Geometry: see drawing. Coordinates: mm, zero at the bounding-box minimum. A direction names the side the tool comes from. Round coordinates to 2 decimals unless told otherwise and drop trailing zeros. Write each loop counter-clockwise with the first axis right and the second up, starting at its lowest first coordinate (ties: lowest second). Pieces come first, ordered by that corner, then holes. Notation, with made-up numbers: M -29.75,39 L -22.75,39 A21 cw -22.75,76 Z; hole C -29,12 d10. An arc over 180 degrees is marked long. Use a Markdown table: item, result.
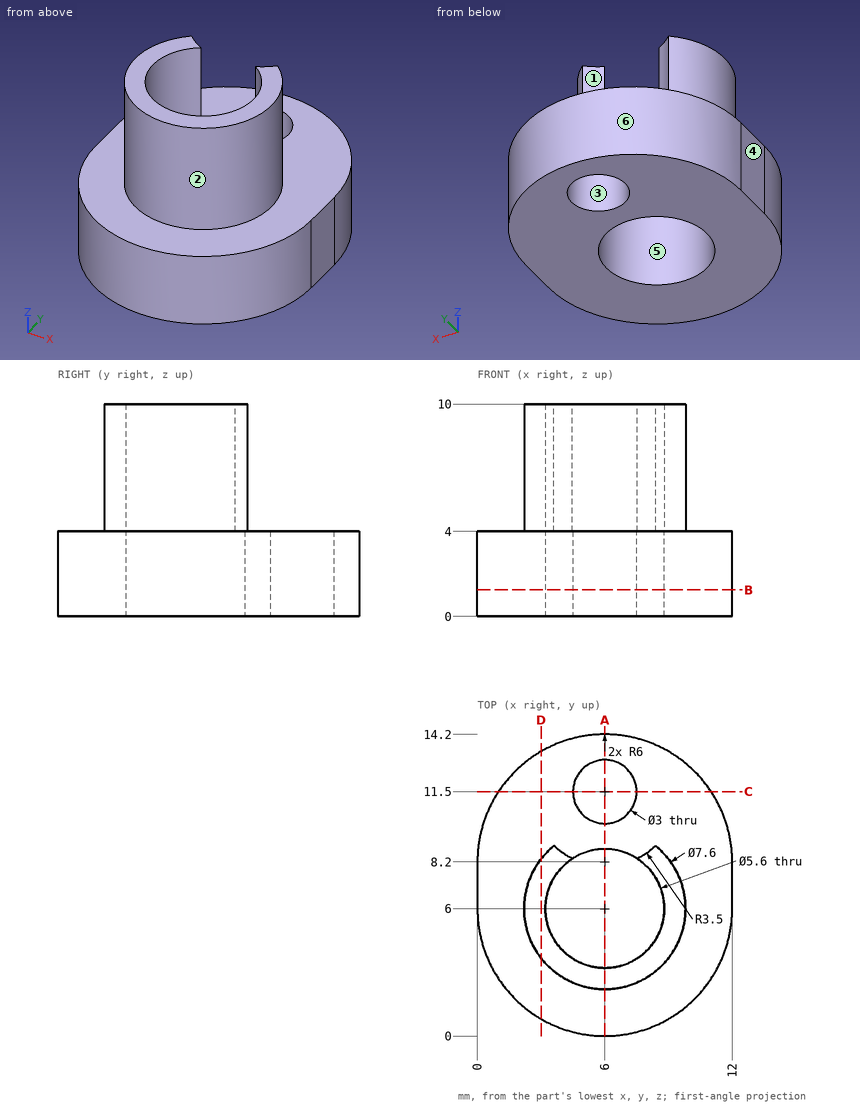
Q1. Section C-C on y = 11.5. Return loops of the section in (x, z).
Results are:
| item | result |
|---|---|
| outline | M 0.99,0 L 4.5,0 L 4.5,4 L 0.99,4 Z; M 7.5,0 L 11.01,0 L 11.01,4 L 7.5,4 Z |
Q2. Section B-B on z = 1.25. Return loops of the section in (x, y).
Results are:
| item | result |
|---|---|
| outline | M 0,6 A6 ccw 12,6 L 12,8.2 A6 ccw 0,8.2 Z; hole C 6,6 d5.6; hole C 6,11.5 d3 |
Q3. Reachability of the marked faces 1, 2 and 3 from +Z, -Z, +X, -X, +Y, -Y: full face, straight path, thin tool, end or side. Return the list, or none.
Results are:
| item | result |
|---|---|
| face 1 | +Z, +Y |
| face 2 | +Z |
| face 3 | +Z, -Z |
Q4. Mould query, pull axis X, two halves, no side actions, for the marked faces 4, 5 and 6. Classes: +X half, -X half, draft (parallel to the pull), parting line (faces both ways), or undercut.
Results are:
| item | result |
|---|---|
| face 4 | -X half |
| face 5 | undercut |
| face 6 | parting line |
Q5. Section D-D on x = 3. Return loops of the section in (y, z), plus the area to 3 significant figures.
Results are:
| item | result |
|---|---|
| outline | M 0.8,0 L 13.4,0 L 13.4,4 L 8.33,4 L 8.33,10 L 3.67,10 L 3.67,4 L 0.8,4 Z |
| area | 78.4 mm^2 |
Q6. Section A-A on x = 6. Return loops of the section in (y, z).
Results are:
| item | result |
|---|---|
| outline | M 0,0 L 3.2,0 L 3.2,10 L 2.2,10 L 2.2,4 L 0,4 Z; M 8.8,0 L 10,0 L 10,4 L 8.8,4 Z; M 13,0 L 14.2,0 L 14.2,4 L 13,4 Z |
Q7. First-contact query: pin 1 Ø6 at (x, y) = (3.5, 2.5) entering from -Z; pin 2 Ø5 at (x, z) = (8.5, 5.5) entering from -Y; pin 3 Ø2 at (x, z) = (7, 6) entering from +Y; pin 4 Ø3 at (x, z) = (8.5, 1.5) entering from -Y. Flat tips, straight axial feed; report the tip coordinate or a pass-through.
Results are:
| item | result |
|---|---|
| pin 1 | z = 0 |
| pin 2 | y = 0.02 |
| pin 3 | y = 8.63 |
| pin 4 | y = 0.08 |
Q8. Line query: L1, parallel to Y at x = 6, z = 2.75; L2, parallel to X at y = 6, z = 5; L3, parallel to Y at x = 6, z = 7.75. Output: solid intervals per line, ascending.
Results are:
| item | result |
|---|---|
| L1 | 0 to 3.2, 8.8 to 10, 13 to 14.2 |
| L2 | 2.2 to 3.2, 8.8 to 9.8 |
| L3 | 2.2 to 3.2 |
